Part model, mm, in its own coordinate system. A direction names the side the tool comes from. Give positions to 0.01 mm unless a question says otherwise; leave off trailing zeros. Order: outer loops, then holes, each group sorted by start corner. A loop starts at its lowest first (then second) coordinate and runs counter-clockwise, first axis right, second up. Notation, with made-up numbers: M 68.5,16.5 L 94.5,16.5 A25 ccw 94.5,52.5 Z; hole C -3,73 d9. An arc over 180 degrees is marked long. One line per question, with ' | ' between items.
```python
from build123d import *

# Parameters (mm, degrees)
BOSS_EXTRUDE1_DEPTH = 160
SKETCH2_W           = 160
SKETCH2_H           = 2
BOSS_EXTRUDE2_DEPTH = 20
BOSS_EXTRUDE3_START = 3
BOSS_EXTRUDE3_DEPTH = 3
SKETCH4_W           = 46.887714477
SKETCH4_H           = 41.449681409
SKETCH4_W_2         = 49.578331284
SKETCH4_H_2         = 39.698074899
SKETCH4_W_3         = 39.67361458
CUT_EXTRUDE1_DEPTH  = 170.375322878


with BuildPart() as part:
    # Sketch1 → Boss-Extrude1 (new body)
    with BuildSketch(Plane(origin=(0, 0, 0), x_dir=(0, 0, -1), z_dir=(1, 0, 0))):
        with BuildLine():
            Line((26, 0), (28, 0))
            ThreePointArc((28, 0), (0, -28), (-28, 0))
            Line((-28, 0), (-26, 0))
            ThreePointArc((-26, 0), (0, -26), (26, 0))
        make_face()
    extrude(amount=BOSS_EXTRUDE1_DEPTH)

    # Sketch2 → Boss-Extrude2 (add)
    with BuildSketch(Plane(origin=(0, 0, 0), x_dir=(1, 0, 0), z_dir=(0, 1, 0))):
        with Locations((80, 27)):
            Rectangle(SKETCH2_W, SKETCH2_H)
        with Locations((80, -27)):
            Rectangle(SKETCH2_W, SKETCH2_H)
    extrude(amount=BOSS_EXTRUDE2_DEPTH)

    # Sketch3 → Boss-Extrude3 (add)
    with BuildSketch(Plane.ZY.offset(BOSS_EXTRUDE3_START)):
        with BuildLine():
            Line((-28, 20), (28, 20))
            Line((28, 20), (28, 0))
            ThreePointArc((28, 0), (0, -28), (-28, 0))
            Line((-28, 0), (-28, 20))
        make_face()
    extrude(amount=-BOSS_EXTRUDE3_DEPTH)

    # Sketch4 → Cut-Extrude1 (cut, through all)
    with BuildSketch(Plane(origin=(0, 20, 0), x_dir=(1, 0, 0), z_dir=(0, 1, 0))):
        with Locations((28.117150866, 1.72863595)):
            Rectangle(SKETCH4_W, SKETCH4_H)
        with Locations((83.472139496, 2.604439205)):
            Rectangle(SKETCH4_W_2, SKETCH4_H_2)
        with Locations((134.499287451, 2.604439205)):
            Rectangle(SKETCH4_W_3, SKETCH4_H_2)
    extrude(amount=-CUT_EXTRUDE1_DEPTH, mode=Mode.SUBTRACT)


solid = part.part
```
1. Tool access for faces 4 (the flat face through (54, 20, 27)), 5 (the flat face through (79, 10, 26)), 6 (the flat face through (28, -19, 18.996)), 7 (the flat face through (83, -15, -22.453)): list every direction of +Z, -Z, +X, -X, +Y, -Y with a clear straight run to the whole face (end or side of a thin tool).
Worked out:
face 4: +Z, -Z, +X, -X, +Y | face 5: +X, +Y | face 6: -Z, +Y, -Y | face 7: +Y, -Y
2. Mould opens along Z. For faces 1 (the cylindrical face through (77.359, -21.048, 18.465)), 2 (the flat face through (79, 10, -26)), 3 (the flat face through (-3, -4, 0)) say: released by +Z, released by -Z, zero draft, split by the parting line, or undercut.
Worked out:
face 1: split by the parting line | face 2: undercut | face 3: zero draft
3. Slice it at B-B on x = 138.5. Give the cut face in (y, z), then the cut area to 3 significant figures.
Worked out:
outline: M -22.06,17.24 L -19.46,17.24 A26 cw 0,26 L 20,26 L 20,28 L 0,28 A28 ccw Z; M -16.73,-22.45 A28 ccw 0,-28 L 20,-28 L 20,-26 L 0,-26 A26 cw -13.11,-22.45 Z | area: 159 mm2
4. Slice it at A-A on z = 0. Give the cut face in (x, y).
Worked out:
outline: M -3,-28 L 4.67,-28 L 4.67,-26 L 0,-26 L 0,20 L -3,20 Z; M 51.56,-28 L 58.68,-28 L 58.68,-26 L 51.56,-26 Z; M 108.26,-28 L 114.66,-28 L 114.66,-26 L 108.26,-26 Z; M 154.34,-28 L 160,-28 L 160,-26 L 154.34,-26 Z
5. Probe L1, parallel to Z at x = 100, y = 16; L2, parallel to X at y = -2.5, z = 20.5; L3, parallel to Z at x = 133, y = -4. List the from-to ranges inside material, lowest first. Write a range as from..to.
Worked out:
L1: z = -28..-26, 26..28 | L2: x = -3..0 | L3: z = -27.71..-25.69, 25.69..27.71
6. Drop flat-ended pins along their axis: pin 1 (7.5 mm diameter, centred on y = -20, z = -5, fed in from +X); pin 2 (6 mm diameter, centred on x = 87.5, z = -20, fed in from +Y); pin 3 (3 mm diameter, centred on x = 126.5, y = -20.5, fed in from -Z); pin 4 (3 mm diameter, centred on x = 124, z = 14, fed in from -Y). Give the stop position or say it passes through.
Worked out:
pin 1: stops at x = 0 | pin 2: stops at y = -12.12 | pin 3: stops at z = 17.24 | pin 4: passes through
7. Slice it at D-D on x = 38. Give the cut face in (y, z).
Worked out:
outline: M -20.57,19 L -17.75,19 A26 cw 0,26 L 20,26 L 20,28 L 0,28 A28 ccw Z; M -16.73,-22.45 A28 ccw 0,-28 L 20,-28 L 20,-26 L 0,-26 A26 cw -13.11,-22.45 Z
8. Slice it at C-C on y = 13. Give the cut face in (x, z), then the cut area to 3 significant figures.
Worked out:
outline: M -3,-28 L 160,-28 L 160,-26 L 0,-26 L 0,26 L 160,26 L 160,28 L -3,28 Z | area: 808 mm2
